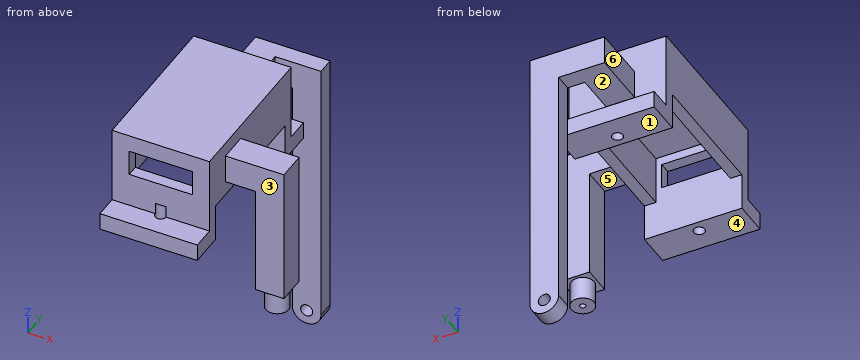
```python
from build123d import *

# Parameters (mm, degrees)
SKETCH1_W            = 4.8
SKETCH1_H            = 4.8
BOSS_EXTRUDE1_DEPTH  = 1
SKETCH2_W            = 5.2
SKETCH2_H            = 5.2
BOSS_EXTRUDE2_DEPTH  = 50
SKETCH3_W            = 17
SKETCH3_H            = 27
BOSS_EXTRUDE3_DEPTH  = 10
SKETCH4_W            = 13
SKETCH4_H            = 23
CUT_EXTRUDE1_DEPTH   = 8.5
SKETCH5_W            = 11
SKETCH5_H            = 4.5
CUT_EXTRUDE2_DEPTH   = 4
SKETCH13_W           = 17
SKETCH13_H           = 27
CUT_EXTRUDE3_DEPTH   = 55.521738784
SKETCH14_W           = 17
SKETCH14_H           = 2
BOSS_EXTRUDE5_DEPTH  = 6.5
SKETCH15_W           = 17
SKETCH15_H           = 3
BOSS_EXTRUDE6_DEPTH  = 4
SKETCH16_R           = 0.95
CUT_EXTRUDE4_DEPTH   = 5
SKETCH17_W           = 5
SKETCH17_H           = 5
BOSS_EXTRUDE7_DEPTH  = 10.2
SKETCH18_W           = 5
SKETCH18_H           = 5
BOSS_EXTRUDE8_DEPTH  = 23.1
SKETCH19_W           = 5
SKETCH19_H           = 5
SKETCH19_R           = 2
CUT_EXTRUDE5_DEPTH   = 4
SKETCH20_R           = 0.5
CUT_EXTRUDE6_DEPTH   = 4
SKETCH21_W           = 5
SKETCH21_H           = 5
BOSS_EXTRUDE9_DEPTH  = 10
SKETCH22_W           = 5
SKETCH22_H           = 3
BOSS_EXTRUDE10_DEPTH = 42.402
SKETCH23_R           = 2.5
BOSS_EXTRUDE11_DEPTH = 3
SKETCH24_R           = 1.05
CUT_EXTRUDE7_DEPTH   = 3
SKETCH26_W           = 13
SKETCH26_H           = 5
BOSS_EXTRUDE12_DEPTH = 3
SKETCH28_W           = 5
SKETCH28_H           = 3
BOSS_EXTRUDE13_DEPTH = 42.402
SKETCH29_R           = 2.5
BOSS_EXTRUDE14_DEPTH = 3
SKETCH30_R           = 1.05
CUT_EXTRUDE8_DEPTH   = 3
SKETCH32_W           = 44.902
SKETCH32_H           = 3
CUT_EXTRUDE9_DEPTH   = 109.298336109


with BuildPart() as part:
    # Sketch1 → Boss-Extrude1 (new body)
    with BuildSketch(Plane.XY):
        with Locations((2.4, -2.4)):
            Rectangle(SKETCH1_W, SKETCH1_H)
    extrude(amount=BOSS_EXTRUDE1_DEPTH)

    # Sketch2 → Boss-Extrude2 (add)
    with BuildSketch(Plane(origin=(0, 0, 0), x_dir=(-1, 0, 0), z_dir=(0, 0, -1))):
        with Locations((-2.4, -2.4)):
            Rectangle(SKETCH2_W, SKETCH2_H)
    extrude(amount=BOSS_EXTRUDE2_DEPTH)

    # Sketch3 → Boss-Extrude3 (add)
    with BuildSketch(Plane(origin=(0, 0, -50), x_dir=(-1, 0, 0), z_dir=(0, 0, -1))):
        with Locations((-2.4, -2.4)):
            Rectangle(SKETCH3_W, SKETCH3_H)
    extrude(amount=BOSS_EXTRUDE3_DEPTH)

    # Sketch4 → Cut-Extrude1 (cut)
    with BuildSketch(Plane(origin=(0, 0, -60), x_dir=(-1, 0, 0), z_dir=(0, 0, -1))):
        with Locations((-2.4, -2.4)):
            Rectangle(SKETCH4_W, SKETCH4_H)
    extrude(amount=-CUT_EXTRUDE1_DEPTH, mode=Mode.SUBTRACT)

    # Sketch5 → Cut-Extrude2 (cut)
    with BuildSketch(Plane.XZ.offset(15.9)):
        with Locations((2.4, -55.25)):
            Rectangle(SKETCH5_W, SKETCH5_H)
    extrude(amount=-CUT_EXTRUDE2_DEPTH, mode=Mode.SUBTRACT)

    # Sketch13 → Cut-Extrude3 (cut, through all)
    with BuildSketch(Plane.XY.offset(-50)):
        with Locations((2.4, -2.4)):
            Rectangle(SKETCH13_W, SKETCH13_H)
    extrude(amount=CUT_EXTRUDE3_DEPTH, mode=Mode.SUBTRACT)

    # Sketch14 → Boss-Extrude5 (add)
    with BuildSketch(Plane(origin=(0, 0, -60), x_dir=(-1, 0, 0), z_dir=(0, 0, -1))):
        with Locations((-2.4, 10.1)):
            Rectangle(SKETCH14_W, SKETCH14_H)
    boss_extrude5 = extrude(amount=BOSS_EXTRUDE5_DEPTH)

    # Sketch15 → Boss-Extrude6 (add)
    with BuildSketch(Plane(origin=(0, 11.1, 0), x_dir=(1, 0, 0), z_dir=(0, 1, 0))):
        with Locations((2.4, 65)):
            Rectangle(SKETCH15_W, SKETCH15_H)
    boss_extrude6 = extrude(amount=BOSS_EXTRUDE6_DEPTH)

    # Sketch16 → Cut-Extrude4 (cut)
    with BuildSketch(Plane(origin=(0, 0, -66.5), x_dir=(-1, 0, 0), z_dir=(0, 0, -1))):
        with Locations((-2.4, 11.1)):
            Circle(SKETCH16_R)
    cut_extrude4 = extrude(amount=-CUT_EXTRUDE4_DEPTH, mode=Mode.SUBTRACT)

    # Mirror2: Boss-Extrude5, Boss-Extrude6, Cut-Extrude4 across plane
    add(boss_extrude5.mirror(Plane(origin=(0, -2.4, 0), x_dir=(0, 0, 1), z_dir=(0, -1, 0))))
    add(boss_extrude6.mirror(Plane(origin=(0, -2.4, 0), x_dir=(0, 0, 1), z_dir=(0, -1, 0))))
    add(cut_extrude4.mirror(Plane(origin=(0, -2.4, 0), x_dir=(0, 0, 1), z_dir=(0, -1, 0))), mode=Mode.SUBTRACT)

    # Sketch17 → Boss-Extrude7 (add)
    with BuildSketch(Plane(origin=(10.9, 0, 0), x_dir=(0, 0, -1), z_dir=(1, 0, 0))):
        with Locations((55, -8.1)):
            Rectangle(SKETCH17_W, SKETCH17_H)
    extrude(amount=BOSS_EXTRUDE7_DEPTH)

    # Sketch18 → Boss-Extrude8 (add)
    with BuildSketch(Plane(origin=(0, 0, -57.5), x_dir=(-1, 0, 0), z_dir=(0, 0, -1))):
        with Locations((-18.6, -8.1)):
            Rectangle(SKETCH18_W, SKETCH18_H)
    extrude(amount=BOSS_EXTRUDE8_DEPTH)

    # Sketch19 → Cut-Extrude5 (cut)
    with BuildSketch(Plane(origin=(0, 0, -80.6), x_dir=(-1, 0, 0), z_dir=(0, 0, -1))):
        with Locations((-18.6, -8.1)):
            Rectangle(SKETCH19_W, SKETCH19_H)
        with Locations((-18.6, -8.1)):
            Circle(SKETCH19_R, mode=Mode.SUBTRACT)
    extrude(amount=-CUT_EXTRUDE5_DEPTH, mode=Mode.SUBTRACT)

    # Sketch20 → Cut-Extrude6 (cut)
    with BuildSketch(Plane(origin=(0, 0, -80.6), x_dir=(-1, 0, 0), z_dir=(0, 0, -1))):
        with Locations((-18.6, -8.1)):
            Circle(SKETCH20_R)
    extrude(amount=-CUT_EXTRUDE6_DEPTH, mode=Mode.SUBTRACT)

    # Sketch21 → Boss-Extrude9 (add)
    with BuildSketch(Plane(origin=(0, 11.1, 0), x_dir=(1, 0, 0), z_dir=(0, 1, 0))):
        with Locations((1.9, 57.5)):
            Rectangle(SKETCH21_W, SKETCH21_H)
    extrude(amount=BOSS_EXTRUDE9_DEPTH)

    # Sketch22 → Boss-Extrude10 (add)
    with BuildSketch(Plane(origin=(0, 0, -60), x_dir=(-1, 0, 0), z_dir=(0, 0, -1))):
        with Locations((-1.9, 19.6)):
            Rectangle(SKETCH22_W, SKETCH22_H)
    extrude(amount=BOSS_EXTRUDE10_DEPTH)

    # Sketch23 → Boss-Extrude11 (add)
    with BuildSketch(Plane(origin=(0, 21.1, 0), x_dir=(1, 0, 0), z_dir=(0, 1, 0))):
        with Locations((1.9, 102.402)):
            Circle(SKETCH23_R)
    extrude(amount=-BOSS_EXTRUDE11_DEPTH)

    # Sketch24 → Cut-Extrude7 (cut)
    with BuildSketch(Plane(origin=(0, 21.1, 0), x_dir=(1, 0, 0), z_dir=(0, 1, 0))):
        with Locations(Location((1.9, 102.402, 0), (0, 0, 270))):
            Circle(SKETCH24_R)
    extrude(amount=-CUT_EXTRUDE7_DEPTH, mode=Mode.SUBTRACT)

    # Sketch26 → Boss-Extrude12 (add)
    with BuildSketch(Plane(origin=(0, 21.1, 0), x_dir=(1, 0, 0), z_dir=(0, 1, 0))):
        with Locations((5.9, 57.5)):
            Rectangle(SKETCH26_W, SKETCH26_H)
    extrude(amount=-BOSS_EXTRUDE12_DEPTH)

    # Sketch28 → Boss-Extrude13 (add)
    with BuildSketch(Plane(origin=(0, 0, -60), x_dir=(-1, 0, 0), z_dir=(0, 0, -1))):
        with Locations((-9.9, 19.6)):
            Rectangle(SKETCH28_W, SKETCH28_H)
    extrude(amount=BOSS_EXTRUDE13_DEPTH)

    # Sketch29 → Boss-Extrude14 (add)
    with BuildSketch(Plane(origin=(0, 21.1, 0), x_dir=(1, 0, 0), z_dir=(0, 1, 0))):
        with Locations((9.9, 102.402)):
            Circle(SKETCH29_R)
    extrude(amount=-BOSS_EXTRUDE14_DEPTH)

    # Sketch30 → Cut-Extrude8 (cut)
    with BuildSketch(Plane(origin=(0, 21.1, 0), x_dir=(1, 0, 0), z_dir=(0, 1, 0))):
        with Locations(Location((9.9, 102.402, 0), (0, 0, 270))):
            Circle(SKETCH30_R)
    extrude(amount=-CUT_EXTRUDE8_DEPTH, mode=Mode.SUBTRACT)

    # Sketch32 → Cut-Extrude9 (cut, through all)
    with BuildSketch(Plane(origin=(4.4, 0, 0), x_dir=(0, 0, -1), z_dir=(1, 0, 0))):
        with Locations((82.451, 19.6)):
            Rectangle(SKETCH32_W, SKETCH32_H)
    extrude(amount=-CUT_EXTRUDE9_DEPTH, mode=Mode.SUBTRACT)


solid = part.part
```
Work out the finished part from the listing and answer in its coordinate system (mm). Face numbers are marked on the shaded views. A direction names the side the tool comes from. Round coordinates to 2 decimals unless told otherwise and drop trailing zeros. Write each loop counter-clockwise with the first axis right and the second up, starting at its lowest first coordinate (ties: lowest second). Pieces come first, ordered by that corner, then holes.
1) Flat-ended cylindrical pins translate along their axes: P1, Ø11, axis at x = -1.5, z = -58.5, coming from the -Y side; P2, Ø4, axis at x = 11, z = -93, coming from the -Y side; P3, Ø1.5, axis at y = 19, z = -89, coming from the +X side; P4, Ø1.5, axis at x = 14.5, y = -8.5, coming from the -Z side. Find the tip coordinate at first contact, or state that the pin passes through.
2) A cutting plane is placed at C-C on y = 4. Determine the outline of the cut face in (x, z), and give its area (3 significant figures).
3) Determine the mould class of the marked faces 1, 2 and 3 for opening direction Z: pulls with the +Z half, pulls with the -Z half, needs draft (parallel to the pull), parting line crosses it, or undercut.
4) Which of the six approach directions +Z, -Z, +X, -X, +Y, -Y give full straight-line access (tool end or side, diameter ignored) to the marked faces 4, 5 and 6?
5) A cutting plane is placed at A-A on x = 2.4. Determine the outline of the cut face in (y, z), and give its area (3 significant figures).
6) A cutting plane is placed at D-D on x = 13. Determine the outline of the cut face in (y, z).
7) Consider probe 1 along Y at (x, z) = (2.4, -64); probe 2 along Y at (x, z) = (9, -55.5); probe 3 along X at (y, z) = (7, -58). Determine where each line is inside the solid, lowest interval first.
8) A cutting plane is placed at B-B on x = 9.9. Determine the outline of the cut face in (y, z).
Entries:
1. P1: stops at y = -19.9
1. P2: stops at y = 18.1
1. P3: stops at x = 12.4
1. P4: stops at z = -57.5
2. outline: (-6.1, -60) - (-4.1, -60) - (-4.1, -51.5) - (8.9, -51.5) - (8.9, -60) - (10.9, -60) - (10.9, -50) - (-6.1, -50) - close
2. area: 59.5 mm2
3. face 1: pulls with the -Z half
3. face 2: undercut
3. face 3: needs draft
4. face 4: -Z, +X, -X, -Y
4. face 5: -Z, -Y
4. face 6: +Z, -X, +Y
5. outline: (-19.9, -66.5) - (-16.85, -66.5) - (-16.85, -63.5) - (-19.9, -63.5) - close; (-15.9, -61.5) - (-14.95, -61.5) - (-14.95, -66.5) - (-13.9, -66.5) - (-13.9, -57.5) - (-15.9, -57.5) - close; (-15.9, -53) - (-13.9, -53) - (-13.9, -51.5) - (9.1, -51.5) - (9.1, -66.5) - (10.15, -66.5) - (10.15, -61.5) - (11.1, -61.5) - (11.1, -60) - (21.1, -60) - (21.1, -55) - (11.1, -55) - (11.1, -50) - (-15.9, -50) - close; (12.05, -66.5) - (15.1, -66.5) - (15.1, -63.5) - (12.05, -63.5) - close
5. area: 150 mm2
6. outline: (-10.6, -57.5) - (-5.6, -57.5) - (-5.6, -52.5) - (-10.6, -52.5) - close
7. probe 1: y = -19.9 to -16.85, -14.95 to -13.9, 9.1 to 10.15, 12.05 to 15.1
7. probe 2: y = -15.9 to 11.1, 18.1 to 21.1
7. probe 3: x = -6.1 to -4.1, 8.9 to 10.9
8. outline: (-19.9, -66.5) - (-13.9, -66.5) - (-13.9, -60) - (9.1, -60) - (9.1, -66.5) - (15.1, -66.5) - (15.1, -63.5) - (11.1, -63.5) - (11.1, -50) - (-15.9, -50) - (-15.9, -63.5) - (-19.9, -63.5) - close; (18.1, -104.9) - (21.1, -104.9) - (21.1, -103.45) - (18.1, -103.45) - close; (18.1, -101.35) - (21.1, -101.35) - (21.1, -55) - (18.1, -55) - close
